Geometry check sheet. Reference: the model listing, model coordinates, mm. Round coordinates to 2 decimals unless told otherwise and drop trailing zeros. Write each loop counter-clockwise with the first axis right and the second up, starting at its lowest first coordinate (ties: lowest second). Pieces come first, ordered by that corner, then holes. Notation, with made-up numbers: (9, 26) -> (13, 26) arc R17 ccw to (13, 40) -> close; hole circle Ø10 at (23, -11.75). An arc over 180 degrees is marked (long way). Put each result on its own line as item: value. Start each with the question number.
from build123d import *

# Parameters (mm, degrees)
SKETCH2_W           = 20
SKETCH2_H           = 20
SKETCH2_W_2         = 16.8
SKETCH2_H_2         = 16.8
BOSS_EXTRUDE1_DEPTH = 210
FILLET1_R           = 2
SKETCH3_W           = 20
SKETCH3_H           = 50
BOSS_EXTRUDE2_DEPTH = 2
SKETCH4_W           = 20
SKETCH4_H           = 3
BOSS_EXTRUDE3_DEPTH = 40
FILLET2_R           = 10
SKETCH5_R           = 5
CUT_EXTRUDE1_DEPTH  = 40
SKETCH6_W           = 20
SKETCH6_H           = 270
BOSS_EXTRUDE4_DEPTH = 2


with BuildPart() as part:
    # Sketch2 → Boss-Extrude1 (new, symmetric)
    with BuildSketch(Plane(origin=(0, 0, 0), x_dir=(0, 0, -1), z_dir=(1, 0, 0))):
        Rectangle(SKETCH2_W, SKETCH2_H)
        Rectangle(SKETCH2_W_2, SKETCH2_H_2, mode=Mode.SUBTRACT)
    extrude(amount=BOSS_EXTRUDE1_DEPTH, both=True)

    # Fillet1
    fillet1_edges = [part.edges().sort_by_distance(p)[0] for p in [
        (0, 8.4, 8.4),
        (0, -8.4, 8.4),
        (0, -8.4, -8.4),
        (0, 8.4, -8.4),
        (0, 10, 10),
        (0, -10, 10),
        (0, -10, -10),
        (0, 10, -10),
    ]]
    fillet(fillet1_edges, radius=FILLET1_R)

    # Sketch3 → Boss-Extrude2 (add)
    with BuildSketch(Plane.XZ.offset(10)):
        with Locations((-198, 0)):
            Rectangle(SKETCH3_W, SKETCH3_H)
        with Locations((198, 0)):
            Rectangle(SKETCH3_W, SKETCH3_H)
    extrude(amount=BOSS_EXTRUDE2_DEPTH)

    # Sketch4 → Boss-Extrude3 (add)
    with BuildSketch(Plane.XZ.offset(12)):
        with Locations((-198, 12.5)):
            Rectangle(SKETCH4_W, SKETCH4_H)
        with Locations((-198, -12.5)):
            Rectangle(SKETCH4_W, SKETCH4_H)
        with Locations((198, 12.5)):
            Rectangle(SKETCH4_W, SKETCH4_H)
        with Locations((198, -12.5)):
            Rectangle(SKETCH4_W, SKETCH4_H)
    extrude(amount=BOSS_EXTRUDE3_DEPTH)

    # Fillet2
    fillet2_edges = [part.edges().sort_by_distance(p)[0] for p in [
        (188, -52, 12.5),
        (208, -52, 12.5),
        (208, -52, -12.5),
        (188, -52, -12.5),
        (-188, -52, 12.5),
        (-188, -52, -12.5),
        (-208, -52, 12.5),
        (-208, -52, -12.5),
    ]]
    fillet(fillet2_edges, radius=FILLET2_R - 0.0001)  # a hair under: the kernel refuses the full size

    # Sketch5 → Cut-Extrude1 (cut)
    with BuildSketch(Plane.XY.offset(14)):
        with Locations((-198, -42)):
            Circle(SKETCH5_R)
        with Locations((198, -42)):
            Circle(SKETCH5_R)
    extrude(amount=-CUT_EXTRUDE1_DEPTH, mode=Mode.SUBTRACT)

    # Sketch6 → Boss-Extrude4 (add)
    with BuildSketch(Plane(origin=(0, 10, 0), x_dir=(1, 0, 0), z_dir=(0, 1, 0))):
        with Locations((0, 50)):
            Rectangle(SKETCH6_W, SKETCH6_H)
    extrude(amount=BOSS_EXTRUDE4_DEPTH)


solid = part.part
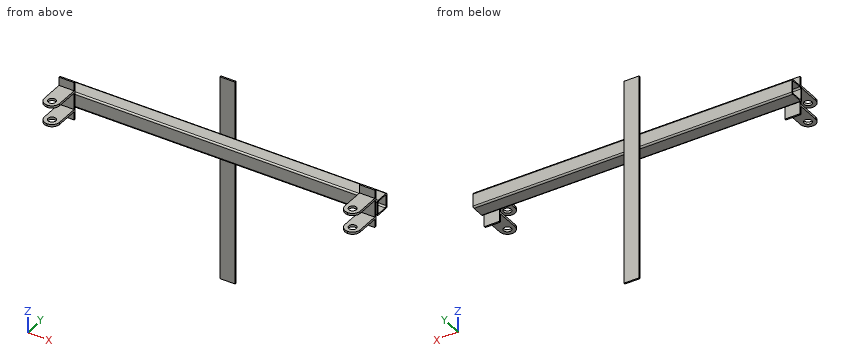
(1) Sectioned sample at C-C (y = -29). Record the cut outline in (x, z), and give its area (3 significant figures).
(2) Sectioned sample at A-A (y = -2). Record the cut outline in (x, z), and give its area (3 significant figures).
(3) Material ranges on L1, parallel to Y at x = -198, z = 13; L2, parallel to Z at x = -193, y = 6; L3, parallel to Y at x = 101.5, z = -9.5, recorded low to high. Write a range as from..to.
(4) Go/stop test with flat-tipped pins: pin 1 Ø9 at (x, z) = (-196, -17) entering from -Y; pin 2 Ø1.6 at (x, z) = (-209, -1) entering from -Y; pin 3 Ø13.5 at (x, z) = (-200.5, 20) entering from +Y; pin 4 Ø10 at (x, y) = (-203, -26.5) entering from -Z. Record where each tip stops, or that it passes through.
(5) Sectioned sample at B-B (x = 100). Record the cut outline in (y, z).
(6) Sectioned sample at D-D (z = -126). Record the cut outline in (x, y).
Found:
1. outline: (-208, -14) -> (-188, -14) -> (-188, -11) -> (-208, -11) -> close; (-208, 11) -> (-188, 11) -> (-188, 14) -> (-208, 14) -> close; (188, -14) -> (208, -14) -> (208, -11) -> (188, -11) -> close; (188, 11) -> (208, 11) -> (208, 14) -> (188, 14) -> close
1. area: 240 mm2
2. outline: (-210, -10) -> (210, -10) -> (210, -8.4) -> (-210, -8.4) -> close; (-210, 8.4) -> (210, 8.4) -> (210, 10) -> (-210, 10) -> close
2. area: 1,340 mm2
3. L1: -52..-47, -37..-10
3. L2: -10..-8.4, 8.4..10
3. L3: -9.32..9.32
4. pin 1: y = -52
4. pin 2: y = -10
4. pin 3: y = -10
4. pin 4: z = -14
5. outline: (-10, -8) arc R2 ccw to (-8, -10) -> (8, -10) arc R2 ccw to (10, -8) -> (10, 8) arc R2 ccw to (8, 10) -> (-8, 10) arc R2 ccw to (-10, 8) -> close; hole (-8.4, -6.4) arc R2 ccw to (-6.4, -8.4) -> (6.4, -8.4) arc R2 ccw to (8.4, -6.4) -> (8.4, 6.4) arc R2 ccw to (6.4, 8.4) -> (-6.4, 8.4) arc R2 ccw to (-8.4, 6.4) -> close
6. outline: (-10, 10) -> (10, 10) -> (10, 12) -> (-10, 12) -> close
